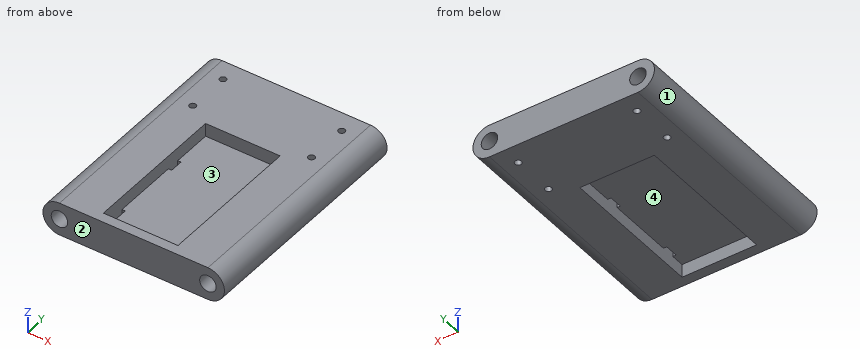
from build123d import *

# Parameters (mm, degrees)
SKETCH2_R           = 3.175
BOSS_EXTRUDE1_DEPTH = 44.45
SKETCH5_R           = 1.27
CUT_EXTRUDE1_DEPTH  = 5.08
CUT_EXTRUDE2_START  = -5.08
SKETCH6_R           = 1.27
CUT_EXTRUDE2_DEPTH  = 5.08
SKETCH7_W           = 28.702
SKETCH7_H           = 55.88
CUT_EXTRUDE3_DEPTH  = 5.08
SKETCH8_W           = 1.27
SKETCH8_H           = 5.08
CUT_EXTRUDE4_DEPTH  = 58.040534053


with BuildPart() as part:
    # Sketch2 → Boss-Extrude1 (new, symmetric)
    with BuildSketch(Plane(origin=(0, 0, 0), x_dir=(1, 0, 0), z_dir=(0, 1, 0))):
        with BuildLine():
            Line((-28.575, 6.35), (28.575, 6.35))
            ThreePointArc((28.575, 6.35), (34.925, 0), (28.575, -6.35))
            Line((28.575, -6.35), (-28.575, -6.35))
            ThreePointArc((-28.575, -6.35), (-34.925, 0), (-28.575, 6.35))
        make_face()
        with Locations(Location((28.575, 0, 0), (0, 0, 270))):
            Circle(SKETCH2_R, mode=Mode.SUBTRACT)
        with Locations(Location((-28.575, 0, 0), (0, 0, 270))):
            Circle(SKETCH2_R, mode=Mode.SUBTRACT)
    extrude(amount=BOSS_EXTRUDE1_DEPTH, both=True)

    # Sketch5 → Cut-Extrude1 (cut)
    with BuildSketch(Plane(origin=(0, 0, -6.35), x_dir=(-1, 0, 0), z_dir=(0, 0, -1))):
        with Locations((22.86, 36.83)):
            Circle(SKETCH5_R)
        with Locations((22.86, 20.32)):
            Circle(SKETCH5_R)
        with Locations((-22.86, 36.83)):
            Circle(SKETCH5_R)
        with Locations((-22.86, 20.32)):
            Circle(SKETCH5_R)
    extrude(amount=-CUT_EXTRUDE1_DEPTH, mode=Mode.SUBTRACT)

    # Sketch6 → Cut-Extrude2 (cut)
    with BuildSketch(Plane.XY.offset(6.35).offset(CUT_EXTRUDE2_START)):
        with Locations(Location((22.86, 36.83, 0), (0, 0, 180))):
            Circle(SKETCH6_R)
        with Locations(Location((22.86, 20.32, 0), (0, 0, 180))):
            Circle(SKETCH6_R)
        with Locations(Location((-22.86, 36.83, 0), (0, 0, 180))):
            Circle(SKETCH6_R)
        with Locations(Location((-22.86, 20.32, 0), (0, 0, 180))):
            Circle(SKETCH6_R)
    extrude(amount=CUT_EXTRUDE2_DEPTH, mode=Mode.SUBTRACT)

    # Sketch7 → Cut-Extrude3 (cut)
    with BuildSketch(Plane.XY.offset(6.35)):
        with Locations((0, -12.7)):
            Rectangle(SKETCH7_W, SKETCH7_H)
    cut_extrude3 = extrude(amount=-CUT_EXTRUDE3_DEPTH, mode=Mode.SUBTRACT)

    # Mirror1: Cut-Extrude3 across plane
    add(cut_extrude3.mirror(Plane.XY), mode=Mode.SUBTRACT)

    # Sketch8 → Cut-Extrude4 (cut, through all)
    with BuildSketch(Plane.XY.offset(1.27)):
        with Locations((13.716, -33.02)):
            Rectangle(SKETCH8_W, SKETCH8_H)
        with Locations((13.716, -2.54)):
            Rectangle(SKETCH8_W, SKETCH8_H)
    cut_extrude4 = extrude(amount=-CUT_EXTRUDE4_DEPTH, mode=Mode.SUBTRACT)

    # Mirror2: Cut-Extrude4 across plane
    add(cut_extrude4.mirror(Plane(origin=(0, 0, 0), x_dir=(0, 0, 1), z_dir=(1, 0, 0))), mode=Mode.SUBTRACT)


solid = part.part
Geometry check sheet. Reference: the model listing, model coordinates, mm. Face numbers are marked on the shaded views. Coordinates: 2 decimals unless noted, no trailing zeros. Order: outer loops, then holes, each group sorted by start corner. A loop starts at its lowest first (then second) coordinate and runs counter-clockwise, first axis right, second up. Notation, with made-up numbers: (89, -34.5) -> (130, -34.5) arc R25 cw to (130, -15.5) -> close; hole circle Ø6 at (78.25, 9). An arc over 180 degrees is marked (long way). Use a Markdown table: item, result. Add a question column.
1. Cross-section at B-B (x = 0.5). Enter the section's corners in (y, z), and give its area (3 significant figures).
2. Go/stop test with flat-tipped pins: pin 1 Ø1 at (y, z) = (-2.5, 1) entering from -X; pin 2 Ø1.5 at (x, y) = (-1.5, -13) entering from +Z. Record where each tip stops, or that it passes through.
3. Mould release check, pull along X, two halves, no side actions. Record for the marked faces 1, 2, 3 and 4: pulls with the +X half, pulls with the -X half, needs draft (parallel to the pull), parting line crosses it, or undercut.
4. Cross-section at C-C (x = -27). Enter the section's corners in (y, z), and give its area (3 significant figures).
5. Cross-section at D-D (z = -5). Enter the section's corners in (x, y).
6. Material ranges on L1, parallel to X at y = 18, z = 0 (3 decimals); L2, parallel to Y at x = 22.86, z = 4.7; L3, parallel to X at y = 34.5, z = 2.25, recorded low to high.
7. Cross-section at A-A (y = 12.5). Enter the section's corners in (x, z) (3 decimals), and give its area (3 significant figures).
Filled sheet:
| question | item | result |
|---|---|---|
| 1 | outline | (-44.45, -6.35) -> (-40.64, -6.35) -> (-40.64, -1.27) -> (15.24, -1.27) -> (15.24, -6.35) -> (44.45, -6.35) -> (44.45, 6.35) -> (15.24, 6.35) -> (15.24, 1.27) -> (-40.64, 1.27) -> (-40.64, 6.35) -> (-44.45, 6.35) -> close |
| 1 | area | 561 mm2 |
| 2 | pin 1 | x = -34.91 |
| 2 | pin 2 | z = 1.27 |
| 3 | face 1 | pulls with the -X half |
| 3 | face 2 | needs draft |
| 3 | face 3 | undercut |
| 3 | face 4 | undercut |
| 4 | outline | (-44.45, -6.35) -> (44.45, -6.35) -> (44.45, -2.76) -> (-44.45, -2.76) -> close; (-44.45, 2.76) -> (44.45, 2.76) -> (44.45, 6.35) -> (-44.45, 6.35) -> close |
| 4 | area | 639 mm2 |
| 5 | outline | (-32.49, -44.45) -> (32.49, -44.45) -> (32.49, 44.45) -> (-32.49, 44.45) -> close; hole circle Ø2.54 at (-22.86, 20.32); hole circle Ø2.54 at (-22.86, 36.83); hole (-14.35, -40.64) -> (14.35, -40.64) -> (14.35, 15.24) -> (-14.35, 15.24) -> close; hole circle Ø2.54 at (22.86, 20.32); hole circle Ø2.54 at (22.86, 36.83) |
| 6 | L1 | -34.925 to -31.75, -25.4 to 25.4, 31.75 to 34.925 |
| 6 | L2 | -44.45 to 19.05, 21.59 to 35.56, 38.1 to 44.45 |
| 6 | L3 | -34.51 to -30.82, -26.33 to 26.33, 30.82 to 34.51 |
| 7 | outline | (-28.575, -6.35) -> (-14.351, -6.35) -> (-14.351, -1.27) -> (14.351, -1.27) -> (14.351, -6.35) -> (28.575, -6.35) arc R6.35 ccw to (28.575, 6.35) -> (14.351, 6.35) -> (14.351, 1.27) -> (-14.351, 1.27) -> (-14.351, 6.35) -> (-28.575, 6.35) arc R6.35 ccw to start; hole circle Ø6.35 at (-28.575, 0); hole circle Ø6.35 at (28.575, 0) |
| 7 | area | 498 mm2 |
